Part model, mm, in its own coordinate system. A direction names the side the tool comes from. Give positions to 0.01 mm unless a question says otherwise; leave off trailing zeros. Write each loop counter-clockwise with the first axis right and the second up, starting at its lowest first coordinate (ties: lowest second). Pieces come first, ordered by that corner, then holes. Notation, with made-up numbers: M 23,-7 L 60,-7 A20 cw 60,16 Z; hole C 9,76 d4. An arc over 180 degrees is marked long. Use a Markdown table: item, result. Add a question column.
from build123d import *

# Parameters (mm, degrees)
SKETCH1_R           = 20
BOSS_EXTRUDE1_DEPTH = 20
SKETCH2_R           = 15
BOSS_EXTRUDE2_DEPTH = 50
SKETCH3_R           = 10
BOSS_EXTRUDE3_DEPTH = 120
SKETCH6_R           = 3
CUT_EXTRUDE1_DEPTH  = 22


with BuildPart() as part:
    # Sketch1 → Boss-Extrude1 (new body)
    with BuildSketch(Plane.XY):
        Circle(SKETCH1_R)
    extrude(amount=BOSS_EXTRUDE1_DEPTH)

    # Sketch2 → Boss-Extrude2 (add)
    with BuildSketch(Plane.XY.offset(20)):
        Circle(SKETCH2_R)
    extrude(amount=BOSS_EXTRUDE2_DEPTH)

    # Sketch3 → Boss-Extrude3 (add)
    with BuildSketch(Plane.XY.offset(70)):
        Circle(SKETCH3_R)
    extrude(amount=BOSS_EXTRUDE3_DEPTH)

    # Sketch5 → Revolve1 (revolve)
    with BuildSketch(Plane(origin=(0, 0, 0), x_dir=(0, 0, -1), z_dir=(1, 0, 0)), mode=Mode.PRIVATE) as revolve1_sk:
        Polygon((-190, 0), (-192, 0), (-192, -8), (-190, -10), align=None)
    revolve(revolve1_sk.sketch.rotate(Axis((0, 0, -30.365330672), (0, 0, 1)), 270), axis=Axis((0, 0, -30.365330672), (0, 0, 1)))

    # Sketch6 → Cut-Extrude1 (cut, symmetric)
    with BuildSketch(Plane(origin=(0, 0, 0), x_dir=(1, 0, 0), z_dir=(0, 1, 0))):
        with Locations(Location((0, -180, 0), (0, 0, 270))):
            Circle(SKETCH6_R)
    extrude(amount=CUT_EXTRUDE1_DEPTH, both=True, mode=Mode.SUBTRACT)


solid = part.part
1. Cut at B-B (x = 0). Write the cut outline in (y, z), then the cut area to 3 significant figures.
2. Tool access for faces 4 (the cylindrical face through (-4.336, -19.524, 9.86)), 5 (the flat face through (3, -10, 70)): list every direction of +Z, -Z, +X, -X, +Y, -Y with a clear straight run to the whole face (end or side of a thin tool).
3. Mould opens along X. For faces 1 (the flat face through (0, 0, 192)), 2 (the conical face through (-7.75, -2.441, 191.875)), 3 (the cylindrical face through (0.9, 0.14, 182.86)) say: released by +X, released by -X, zero draft, split by the parting line, or undercut.
4. Cut at A-A (y = 0). Write the cut outline in (x, z), then the cut area to 3 significant figures.
5. Flat gauge pins, fed straight in: pin 1 (6 mm diameter, centred on x = 2.5, z = 140.5, fed in from +Y); pin 2 (5 mm diameter, centred on y = -4, z = 92.5, fed in from -X); pin 3 (10 mm diameter, centred on x = -12, z = 132, fed in from -Y). Where does each tip first touch, or does it go through?
6. Drill centre lines: probe 1 along X at (y, z) = (0.25, 180); probe 2 along X at (y, z) = (-6, 180); probe 3 along Z at (x, y) = (0, 2.25). Where is each one in solid material? Low to high. Write a range as [from, to].
7. Cut at C-C (z = 24.5). Write the cut outline in (x, y).
8. Cut at D-D (z = 180). Write the cut outline in (x, y), then the cut area to 3 significant figures.
A:
| question | item | result |
|---|---|---|
| 1 | outline | M -20,0 L 20,0 L 20,20 L 15,20 L 15,70 L 10,70 L 10,177 L -10,177 L -10,70 L -15,70 L -15,20 L -20,20 Z; M -10,183 L 10,183 L 10,190 L 8,192 L -8,192 L -10,190 Z |
| 1 | area | 4,620 mm² |
| 2 | face 4 | +Z, -Z |
| 2 | face 5 | +Z |
| 3 | face 1 | zero draft |
| 3 | face 2 | split by the parting line |
| 3 | face 3 | undercut |
| 4 | outline | M -20,0 L 20,0 L 20,20 L 15,20 L 15,70 L 10,70 L 10,190 L 8,192 L -8,192 L -10,190 L -10,70 L -15,70 L -15,20 L -20,20 Z; hole C 0,180 d6 |
| 4 | area | 4,710 mm² |
| 5 | pin 1 | stops at y = 10 |
| 5 | pin 2 | stops at x = -9.89 |
| 5 | pin 3 | stops at y = -7.14 |
| 6 | probe 1 | x = [-10, -3], [3, 10] |
| 6 | probe 2 | x = [-8, -3], [3, 8] |
| 6 | probe 3 | z = [0, 177], [183, 192] |
| 7 | outline | C 0,0 d30 |
| 8 | outline | M -3,-9.54 L -3,9.54 A10 ccw Z; M 3,-9.54 A10 ccw 3,9.54 Z |
| 8 | area | 196 mm² |
